Geometry: final body of the model. Coordinates: model frame, mm. Round coordinates to 2 decimals unless told otherwise and drop trailing zeros. Loops run counter-clockwise (first coordinate to the right, second up) from the corner with the lowest first, then second, coordinate; pieces in that order, holes last. Notation, with made-up numbers: M 62.25,28.5 L 77.25,28.5 A25 ccw 77.25,51.5 Z; hole C -8.5,80 d4. An arc over 180 degrees is marked long. Answer as a JSON object with one key per item and string values.
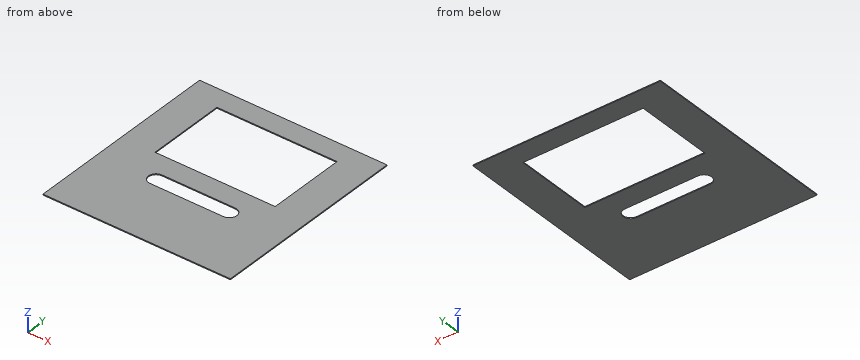
```python
from build123d import *

# Parameters (mm, degrees)
SKETCH1_W           = 382
SKETCH1_H           = 405
BOSS_EXTRUDE1_DEPTH = 2
CUT_EXTRUDE1_DEPTH  = 296.144032635
SKETCH3_W           = 267
SKETCH3_H           = 157
BOSS_EXTRUDE2_DEPTH = 15
SKETCH4_W           = 261
SKETCH4_H           = 151
CUT_EXTRUDE2_DEPTH  = 15
SKETCH5_W           = 245
SKETCH5_H           = 160
CUT_EXTRUDE3_DEPTH  = 296.51818895
SKETCH7_W           = 15
SKETCH7_H           = 157
CUT_EXTRUDE4_DEPTH  = 395.657042985
BOSS_EXTRUDE3_START = -2
BOSS_EXTRUDE3_DEPTH = 2
CUT_EXTRUDE5_DEPTH  = 296.144032635


with BuildPart() as part:
    # Sketch1 → Boss-Extrude1 (new body)
    with BuildSketch(Plane(origin=(0, 0, 0), x_dir=(-1, 0, 0), z_dir=(0, 0, -1))):
        with Locations((0, 22.5)):
            Rectangle(SKETCH1_W, SKETCH1_H)
    extrude(amount=-BOSS_EXTRUDE1_DEPTH)

    # Sketch2 → Cut-Extrude1 (cut, through all)
    with BuildSketch(Plane.XY.offset(2)):
        with BuildLine():
            Line((-75.5, -35.65), (75.482536693, -35.65))
            ThreePointArc((75.482536693, -35.65), (60.004590726, -20), (75.482536693, -4.35))
            Line((75.482536693, -4.35), (-75.5, -4.35))
            ThreePointArc((-75.5, -4.35), (-91.15, -20), (-75.5, -35.65))
        make_face()
    extrude(amount=-CUT_EXTRUDE1_DEPTH, mode=Mode.SUBTRACT)

    # Sketch3 → Boss-Extrude2 (add)
    with BuildSketch(Plane(origin=(0, 0, 0), x_dir=(-1, 0, 0), z_dir=(0, 0, -1))):
        with Locations((-0.610849862, 98.314505171)):
            Rectangle(SKETCH3_W, SKETCH3_H)
    extrude(amount=BOSS_EXTRUDE2_DEPTH)

    # Sketch4 → Cut-Extrude2 (cut)
    with BuildSketch(Plane(origin=(0, 0, -15), x_dir=(-1, 0, 0), z_dir=(0, 0, -1))):
        with Locations((-0.610849862, 98.314505171)):
            Rectangle(SKETCH4_W, SKETCH4_H)
    extrude(amount=-CUT_EXTRUDE2_DEPTH, mode=Mode.SUBTRACT)

    # Sketch5 → Cut-Extrude3 (cut, through all)
    with BuildSketch(Plane(origin=(0, 0, 0), x_dir=(-1, 0, 0), z_dir=(0, 0, -1))):
        with Locations((0, 102.814505171)):
            Rectangle(SKETCH5_W, SKETCH5_H)
    extrude(amount=-CUT_EXTRUDE3_DEPTH, mode=Mode.SUBTRACT)

    # Sketch7 → Cut-Extrude4 (cut, through all)
    with BuildSketch(Plane.ZY.offset(132.889150138)):
        with Locations((-7.5, 98.314505171)):
            Rectangle(SKETCH7_W, SKETCH7_H)
    extrude(amount=-CUT_EXTRUDE4_DEPTH, mode=Mode.SUBTRACT)

    # Sketch9 → Boss-Extrude3 (add)
    with BuildSketch(Plane(origin=(0, 0, 0), x_dir=(-1, 0, 0), z_dir=(0, 0, -1)).offset(BOSS_EXTRUDE3_START)):
        with BuildLine():
            Line((75.5, -35.65), (-75.482536693, -35.65))
            ThreePointArc((-75.482536693, -35.65), (-60.004590726, -20), (-75.482536693, -4.35))
            Line((-75.482536693, -4.35), (75.5, -4.35))
            ThreePointArc((75.5, -4.35), (91.15, -20), (75.5, -35.65))
        make_face()
    extrude(amount=BOSS_EXTRUDE3_DEPTH)

    # Sketch8 → Cut-Extrude5 (cut, through all)
    with BuildSketch(Plane(origin=(0, 0, 0), x_dir=(-1, 0, 0), z_dir=(0, 0, -1))):
        with BuildLine():
            Line((-73.827773505, -20), (73.827773505, -20))
            ThreePointArc((73.827773505, -20), (89.945940018, -35.25), (73.827773505, -50.5))
            Line((73.827773505, -50.5), (-73.827773505, -50.5))
            ThreePointArc((-73.827773505, -50.5), (-89.945940018, -35.25), (-73.827773505, -20))
        make_face()
    extrude(amount=-CUT_EXTRUDE5_DEPTH, mode=Mode.SUBTRACT)


solid = part.part
```
1) Cut plane B-B on y = -35.25. Return the cut outline in (x, z).
Geometry results:
{"outline": "M -191,0 L -89.95,0 L -89.95,2 L -191,2 Z; M 89.95,0 L 191,0 L 191,2 L 89.95,2 Z"}
2) Cut plane D-D on y = 136.5. Return the cut outline in (x, z).
Geometry results:
{"outline": "M -191,0 L -122.5,0 L -122.5,2 L -191,2 Z; M 122.5,0 L 191,0 L 191,2 L 122.5,2 Z"}
3) Cut plane C-C on z = 1.15. Return the cut outline in (x, y), and give its area (3 significant figures).
Geometry results:
{"outline": "M -191,-180 L 191,-180 L 191,225 L -191,225 Z; hole M -122.5,22.81 L 122.5,22.81 L 122.5,182.81 L -122.5,182.81 Z; hole M -73.83,-50.5 L 73.83,-50.5 A15.27 ccw long 73.83,-20 L -73.83,-20 A15.27 ccw long Z", "area": "110,000 mm2"}
4) Cut plane A-A on x = 56. Return the cut outline in (y, z).
Geometry results:
{"outline": "M -180,0 L -50.5,0 L -50.5,2 L -180,2 Z; M -20,0 L 22.81,0 L 22.81,2 L -20,2 Z; M 182.81,0 L 225,0 L 225,2 L 182.81,2 Z"}
5) Line query: probe 1 along Y at (x, z) = (-48, 0.4); probe 2 along X at (y, z) = (143, 0.35); probe 3 along Y at (x, z) = (116.5, 0.35). Output: solid intervals per line, ascending.
Geometry results:
{"probe 1": "-180 to -50.5, -20 to 22.81, 182.81 to 225", "probe 2": "-191 to -122.5, 122.5 to 191", "probe 3": "-180 to 22.81, 182.81 to 225"}
